Check sheet for the modelled part. Datum: model origin and axes. Units: mm. Face numbers are marked on the shaded views. Round coordinates to 2 decimals unless told otherwise and drop trailing zeros. Loops run counter-clockwise (first coordinate to the right, second up) from the corner with the lowest first, then second, coordinate; pieces in that order, holes last. Notation, with made-up numbers: (48.5, -33) -> (72.5, -33) arc R30 ccw to (72.5, -7) -> close; hole circle Ø2 at (47.5, 77.25). An arc over 180 degrees is marked (long way). Use one line per item in the form item = value. Start each with the question number.
(1) Sectioned sample at B-B (x = 0). Record the cut outline in (y, z), and give its area (3 significant figures).
(2) Material ranges on probe 1 along Z at (x, y) = (0, 51); probe 2 along Z at (x, y) = (3, 107); probe 3 along X at (y, z) = (62.5, -32), recorded low to high. Write a range as [from, to].
(3) Sectioned sample at A-A (z = 0). Record the cut outline in (x, y).
(4) Go/stop test with flat-tipped pins: pin 1 (9 mm diameter, centred on x = 0, z = -47.5, fed in from -Y); pin 2 (2 mm diameter, centred on x = -39, y = 94, fed in from +Z); pin 3 (4 mm diameter, centred on x = -34.5, y = 23, fed in from -Z); pin 4 (5 mm diameter, centred on x = 17.5, y = 76.5, fed in from -Z) (3 decimals). Record where each tip stops, or that it passes through.
(5) Draft check along Z on the marked faces 1, 2 and 3. Enter one of: released by +Z, released by -Z, zero draft, split by the parting line, or undercut.
(6) Sectioned sample at C-C (z = 27). Record the cut outline in (x, y), and give its area (3 significant figures).
(7) Sectioned sample at D-D (x = 47.5). Record the cut outline in (y, z).
Autodesk Inventor part; units mm, degrees
ref_plane "YZ Plane" through (0, 0, 0) normal (1, 0, 0) x (0, 1, 0)
ref_plane "XZ Plane" through (0, 0, 0) normal (0, 1, 0) x (-1, 0, 0)
ref_plane "XY Plane" through (0, 0, 0) normal (0, 0, 1) x (1, 0, 0)
sketch "Sketch1" plane through (0, 0, 0) normal (0, 1, 0) x (-1, 0, 0)
  circle A0 centre (0, 0) radius 40
  circle A1 centre (0, 0) radius 55
  circle A2 centre (47.5, 0) radius 5.5
  circle A3 centre (0, -47.5) radius 5.5
  circle A4 centre (0, 47.5) radius 5.5
  circle A5 centre (-47.5, 0) radius 5.5
  dimension "d0" = 80
  dimension "d10" = 11
  dimension "d11" = 11
  dimension "d12" = 11
  dimension "d13" = 11
extrude "Extrusion1" add sketch "Sketch1" along normal blind 120
equation "\"BendRadius\" = Thickness"
equation "\"BendReliefWidth\" = Thickness"
equation "\"BendReliefDepth\" = 0.5 * Thickness"
equation "\"CornerReliefSize\" = 4 * Thickness"
equation "\"MinimumRemnant\" = 2 * Thickness"
equation "\"TransitionRadius\" = BendRadius"
equation "\"JacobiRadiusSize\" = BendRadius"
equation "\"GapSize\" = Thickness"
properties part number "cilindro"
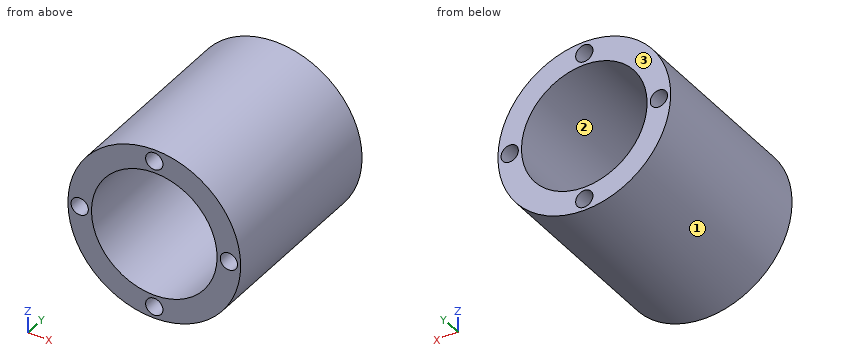
Checks:
q1.outline = (0, -55) -> (120, -55) -> (120, -53) -> (0, -53) -> close; (0, -42) -> (120, -42) -> (120, -40) -> (0, -40) -> close; (0, 40) -> (120, 40) -> (120, 42) -> (0, 42) -> close; (0, 53) -> (120, 53) -> (120, 55) -> (0, 55) -> close
q1.area = 960 mm2
q2.probe_1 = [-55, -53], [-42, -40], [40, 42], [53, 55]
q2.probe_2 = [-54.92, -52.11], [-42.89, -39.89], [39.89, 42.89], [52.11, 54.92]
q2.probe_3 = [-44.73, -24], [24, 44.73]
q3.outline = (-55, 0) -> (-53, 0) -> (-53, 120) -> (-55, 120) -> close; (-42, 0) -> (-40, 0) -> (-40, 120) -> (-42, 120) -> close; (40, 0) -> (42, 0) -> (42, 120) -> (40, 120) -> close; (53, 0) -> (55, 0) -> (55, 120) -> (53, 120) -> close
q4.pin_1 = through
q4.pin_2 = 39.76
q4.pin_3 = -44.37
q4.pin_4 = -52.915
q5.face_1 = split by the parting line
q5.face_2 = undercut
q5.face_3 = zero draft
q6.outline = (-47.92, 0) -> (-29.51, 0) -> (-29.51, 120) -> (-47.92, 120) -> close; (29.51, 0) -> (47.92, 0) -> (47.92, 120) -> (29.51, 120) -> close
q6.area = 4,420 mm2
q7.outline = (0, -27.73) -> (120, -27.73) -> (120, -5.5) -> (0, -5.5) -> close; (0, 5.5) -> (120, 5.5) -> (120, 27.73) -> (0, 27.73) -> close
